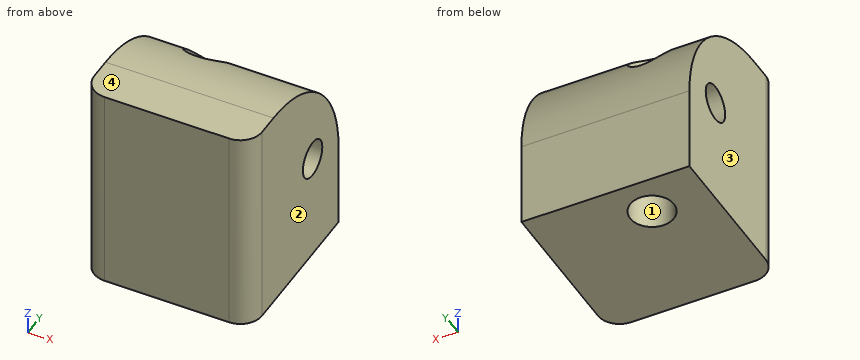
```python
from build123d import *

# Parameters (mm, degrees)
F0_R        = 6.5
F1_DEPTH    = 63
F2_T1_DEPTH = 235.8944443027
F3_R        = 5.5443537003
F4_DEPTH    = 50.0010001


# Not quite as in the source:
# - a fillet or chamfer that OpenCascade refuses, or shapes differently, is made with other operations: its cross-section is extruded or revolved along the edge and cut away or added


with BuildPart() as f1:
    # F0 (on Top) → F1 (new body)
    with BuildSketch(Plane.XY):
        with BuildLine():
            ThreePointArc((-25, -18.57671062), (-23.1040174372, -23.1540174372), (-18.52671062, -25.05))
            Line((-18.52671062, -25.05), (18.52671062, -25.05))
            ThreePointArc((18.52671062, -25.05), (23.1040174372, -23.1540174372), (25, -18.57671062))
            Line((25, -18.57671062), (25, 25.05))
            Line((25, 25.05), (-25, 25.05))
            Line((-25, 25.05), (-25, -18.57671062))
        make_face()
        with Locations((-7.6206641026, 13.05)):
            Circle(F0_R, mode=Mode.SUBTRACT)
    extrude(amount=F1_DEPTH)

    # F2: fillet of radius 37.1788888605 on 1 edges, made by hand

    # F2_s2 → F2_t1 (cut)
    with BuildSketch(Plane.YZ.offset(-117.9472221514)):
        with BuildLine():
            ThreePointArc((25.05, 25.8211111395), (14.1605555697, 52.1105555697), (-12.1288888605, 63))
            Line((-12.1288888605, 63), (25.05, 63))
            Line((25.05, 63), (25.05, 25.8211111395))
        make_face()
    extrude(amount=F2_T1_DEPTH, mode=Mode.SUBTRACT)

    # F3 (on face) → F4 (cut, through all)
    with BuildSketch(Plane.YZ.offset(25)):
        with Locations((10.2042127401, 32.5643420219)):
            Circle(F3_R)
    extrude(amount=-F4_DEPTH, mode=Mode.SUBTRACT)


solid = f1.part
```
Can you work these out from the model? Positions are in its coordinate system, mm. Face numbers are marked on the shaded views. Coordinates: 2 decimals unless noted, no trailing zeros. Loops run counter-clockwise (first coordinate to the right, second up) from the corner with the lowest first, then second, coordinate; pieces in that order, holes last. Notation, with made-up numbers: (85, 74) -> (122, 74) arc R18 cw to (122, 82) -> close; hole circle Ø8 at (35.25, -17). An arc over 180 degrees is marked (long way). Put each result on its own line as item: value. Start each with the question number.
Q1. Thinking about a two-plate mould opening in X: for the marked faces 1, 2, 3 and 4, which applies, pulls with the +X half, pulls with the -X half, needs draft (parallel to the pull), parting line crosses it, or undercut?
Q2. I want a section at D-D (x = -11.5). Write out the boundary of the cut face in (y, z), plus the area to 3 significant figures.
Q3. I want a section at B-B (x = -5). Write out the boundary of the cut face in (y, z).
Q4. I'm going to push flat-ended pins straight in: P1, Ø2, axis at x = -14, y = -2.5, coming from the -Z side; P2, Ø2, axis at x = -13, y = -4, coming from the +Z side; P3, Ø1.5, axis at x = 9, y = 4.5, coming from the +Z side; P4, Ø6, axis at x = -16.5, z = 56.5, coming from the +Y side. Where does each tip first touch, or does it pass through?
Q5. I want a section at C-C (x = 6.5). Write out the boundary of the cut face in (y, z).
Q6. I want a section at A-A (y = 13.05). Write out the boundary of the cut face in (x, z).
Q7. If I drill on line 1 (X direction, y = 13, z = 23); line 2 (Z direction, x = -13, y = 7); line 3 (Y direction, x = 5, z = 26), over which ranges is the centre line in solid material (lowest first)? Write a range as [from, to].
Taken from the geometry:
1. face 1: undercut
1. face 2: pulls with the +X half
1. face 3: pulls with the -X half
1. face 4: needs draft
2. outline: (-25.05, 0) -> (7.83, 0) -> (7.83, 27.55) arc R5.54 cw to (7.83, 37.58) -> (7.83, 57.19) arc R37.18 ccw to (-12.13, 63) -> (-25.05, 63) -> close; (18.27, 0) -> (25.05, 0) -> (25.05, 25.82) arc R37.18 ccw to (18.27, 47.23) -> close
2. area: 2,290 mm2
3. outline: (-25.05, 0) -> (7.1, 0) -> (7.1, 27.97) arc R5.54 cw to (7.1, 37.16) -> (7.1, 57.64) arc R37.18 ccw to (-12.13, 63) -> (-25.05, 63) -> close; (19, 0) -> (25.05, 0) -> (25.05, 25.82) arc R37.18 ccw to (19, 46.15) -> close
4. P1: stops at z = 0
4. P2: stops at z = 62.31
4. P3: stops at z = 59.44
4. P4: stops at y = 12.69
5. outline: (-25.05, 0) -> (25.05, 0) -> (25.05, 25.82) arc R37.18 ccw to (-12.13, 63) -> (-25.05, 63) -> close; hole circle Ø11.09 at (10.2, 32.56)
6. outline: (-25, 0) -> (-14.12, 0) -> (-14.12, 27.81) -> (-25, 27.81) -> close; (-25, 37.32) -> (-14.12, 37.32) -> (-14.12, 53.18) -> (-25, 53.18) -> close; (-1.12, 0) -> (25, 0) -> (25, 27.81) -> (-1.12, 27.81) -> close; (-1.12, 37.32) -> (25, 37.32) -> (25, 53.18) -> (-1.12, 53.18) -> close
7. line 1: x = [-25, -14.12], [-1.12, 25]
7. line 2: z = [0, 28.04], [37.09, 57.7]
7. line 3: y = [-25.05, 25.05]
